Read the model definition and answer for the solid it produces. Units are mm, in the model's axes. Face numbers are marked on the shaded views. A direction names the side the tool comes from. Round coordinates to 2 decimals unless told otherwise and drop trailing zeros. Loops run counter-clockwise (first coordinate to the right, second up) from the corner with the lowest first, then second, coordinate; pieces in that order, holes last. Notation, with made-up numbers: (35, 4) - (81, 4) arc R5 cw to (81, 8) - close; hole circle Ø8 at (-25.5, -9). An arc over 180 degrees is marked (long way). Answer as CSV lines item,"result".
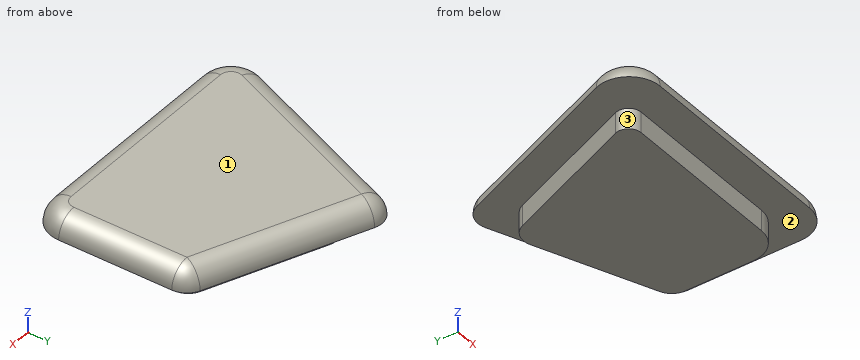
```python
from build123d import *

# Parameters (mm, degrees)
BOSS_EXTRUDE1_DEPTH = 5
BOSS_EXTRUDE2_DEPTH = 5
FILLET1_R           = 5


with BuildPart() as part:
    # Sketch1 → Boss-Extrude1 (new body)
    # profile 1 of 3: a face of its own
    with BuildSketch(Plane.XY):
        with BuildLine():
            Line((32.146013204, 7.5), (32.146013204, 34.934018325))
            ThreePointArc((32.146013204, 34.934018325), (31.303361266, 37.71186949), (29.059430366, 39.553415988))
            Line((29.059430366, 39.553415988), (-7.718495765, 54.787331787))
            ThreePointArc((-7.718495765, 54.787331787), (-11.545330089, 54.787331787), (-14.25131059, 52.081351287))
            Line((-14.25131059, 52.081351287), (-31.528665913, 10.370125743))
            ThreePointArc((-31.528665913, 10.370125743), (-30.835591512, 3.333223252), (-24.599569419, 0))
            Line((-24.599569419, 0), (24.646013204, 0))
            ThreePointArc((24.646013204, 0), (29.949314063, 2.196699141), (32.146013204, 7.5))
        make_face()
        with BuildLine():
            ThreePointArc((27.146013204, 31.593125136), (26.303361266, 34.370976301), (24.059430366, 36.212522798))
            Line((24.059430366, 36.212522798), (-3.230262498, 47.516283695))
            ThreePointArc((-3.230262498, 47.516283695), (-7.057096821, 47.516283695), (-9.763077322, 44.810303195))
            Line((-9.763077322, 44.810303195), (-23.212969116, 12.339392013))
            ThreePointArc((-23.212969116, 12.339392013), (-22.889534395, 9.055504184), (-19.979390752, 7.5))
            Line((-19.979390752, 7.5), (19.646013204, 7.5))
            ThreePointArc((19.646013204, 7.5), (24.949314063, 9.696699141), (27.146013204, 15))
            Line((27.146013204, 15), (27.146013204, 31.593125136))
        make_face(mode=Mode.SUBTRACT)
    # profile 2 of 3: a face of its own
    with BuildSketch(Plane.XY):
        with BuildLine():
            Line((27.146013204, 31.593125136), (27.146013204, 15))
            ThreePointArc((27.146013204, 15), (24.949314063, 9.696699141), (19.646013204, 7.5))
            Line((19.646013204, 7.5), (-19.979390752, 7.5))
            ThreePointArc((-19.979390752, 7.5), (-22.889534395, 9.055504184), (-23.212969116, 12.339392013))
            Line((-23.212969116, 12.339392013), (-9.763077322, 44.810303195))
            ThreePointArc((-9.763077322, 44.810303195), (-7.057096821, 47.516283695), (-3.230262498, 47.516283695))
            Line((-3.230262498, 47.516283695), (24.059430366, 36.212522798))
            ThreePointArc((24.059430366, 36.212522798), (26.303361266, 34.370976301), (27.146013204, 31.593125136))
        make_face()
    # profile 3 of 3: a face of its own
    with BuildSketch(Plane.XY):
        with BuildLine():
            Line((26.646013204, 31.593125136), (26.646013204, 15))
            ThreePointArc((26.646013204, 15), (24.595760673, 10.050252532), (19.646013204, 8))
            Line((19.646013204, 8), (-19.979390752, 8))
            ThreePointArc((-19.979390752, 8), (-22.473799589, 9.333289301), (-22.75102935, 12.148050297))
            Line((-22.75102935, 12.148050297), (-9.301137556, 44.618961479))
            ThreePointArc((-9.301137556, 44.618961479), (-6.865755105, 47.054343929), (-3.421604214, 47.054343929))
            Line((-3.421604214, 47.054343929), (23.86808865, 35.750583032))
            ThreePointArc((23.86808865, 35.750583032), (25.88762646, 34.093191184), (26.646013204, 31.593125136))
        make_face()
    extrude(amount=BOSS_EXTRUDE1_DEPTH)

    # Sketch1<4> → Boss-Extrude2 (add)
    with BuildSketch(Plane.XY):
        with BuildLine():
            Line((26.646013204, 31.593125136), (26.646013204, 15))
            ThreePointArc((26.646013204, 15), (24.595760673, 10.050252532), (19.646013204, 8))
            Line((19.646013204, 8), (-19.979390752, 8))
            ThreePointArc((-19.979390752, 8), (-22.473799589, 9.333289301), (-22.75102935, 12.148050297))
            Line((-22.75102935, 12.148050297), (-9.301137556, 44.618961479))
            ThreePointArc((-9.301137556, 44.618961479), (-6.865755105, 47.054343929), (-3.421604214, 47.054343929))
            Line((-3.421604214, 47.054343929), (23.86808865, 35.750583032))
            ThreePointArc((23.86808865, 35.750583032), (25.88762646, 34.093191184), (26.646013204, 31.593125136))
        make_face()
    extrude(amount=-BOSS_EXTRUDE2_DEPTH)

    # Fillet1
    fillet1_edges = [part.edges().sort_by_distance(p)[0] for p in [
        (29.949314063, 2.196699141, 5),
        (0.023221893, 0, 5),
        (-30.835591512, 3.333223252, 5),
        (-22.889988251, 31.225738515, 5),
        (-11.545330089, 54.787331787, 5),
        (10.670467301, 47.170373888, 5),
        (31.303361266, 37.71186949, 5),
        (32.146013204, 21.217009163, 5),
    ]]
    fillet(fillet1_edges, radius=FILLET1_R - 0.0001)  # a hair under: the kernel refuses the full size


solid = part.part
```
1) Find the intervals of material crossed by line 1 (Z direction, x = 27.5, y = 14.5); line 2 (X direction, y = 27.5, z = -1.75); line 3 (X direction, y = 6, z = 0.5), in increasing order.
Entries:
line 1,"z = 0 to 4.99"
line 2,"x = -16.39 to 26.65"
line 3,"x = -31.92 to 31.97"
2) A tool of negligible diameter and unlimited length cuts with its end or side. For the marked faces 1, 2 and 3, from which of +Z, -Z, +X, -X, +Y, -Y can it reach the whole face along a straight path? Write none if from no direction.
Entries:
face 1,"+Z, +X, -X, +Y, -Y"
face 2,"-Z"
face 3,"-Z, -X"
3) A cutting plane is placed at A-A, the plane z = -1.25. Determine the outline of the cut face in (x, y), plus the area to 3 significant figures.
Entries:
outline,"(-22.75, 12.15) arc R3 ccw to (-19.98, 8) - (19.65, 8) arc R7 ccw to (26.65, 15) - (26.65, 31.59) arc R4.5 ccw to (23.87, 35.75) - (-3.42, 47.05) arc R4.5 ccw to (-9.3, 44.62) - close"
area,"1,480 mm^2"
4) Each of these flat-tipped pins is pushed along its axis until it touches: P1, Ø8, axis at x = -24.5, y = 27, coming from the -Z side; P2, Ø2.5, axis at y = 24, z = -2.5, coming from the +X side; P3, Ø2.5, axis at x = 8, z = -2.5, coming from the -Y side. Where does it stop, or does it pass through?
Entries:
P1,"stops at z = 0"
P2,"stops at x = 26.65"
P3,"stops at y = 8"
